Could you check a few things on this model? Use its own coordinates, in mm. Face numbers are marked on the shaded views. A direction names the side the tool comes from. Coordinates: 2 decimals unless noted, no trailing zeros. Loops run counter-clockwise (first coordinate to the right, second up) from the corner with the lowest first, then second, coordinate; pieces in that order, holes last. Notation, with made-up numbers: (49.5, -32) - (101.5, -32) arc R24 cw to (101.5, 4) - close; hole circle Ø9 at (29.25, 66.5). An arc over 180 degrees is marked (long way). Use CSV: the item, a comma, the result in double quotes.
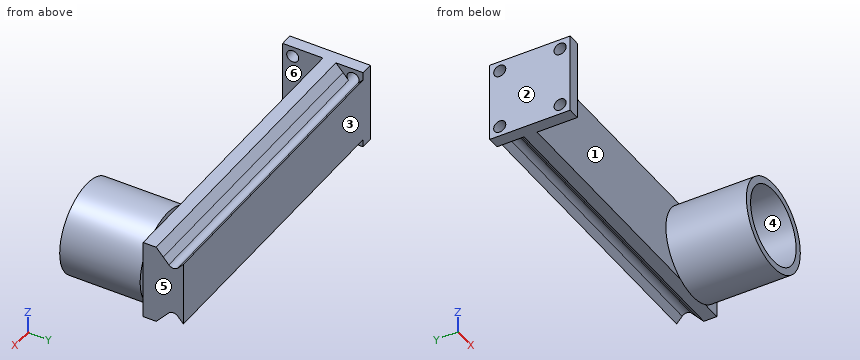
Autodesk Inventor part; units mm, degrees
ref_plane "Work Plane4" through (0, 0, 20) normal (0, 0, -1) x (1, 0, 0)
ref_plane "YZ Plane" through (0, 0, 0) normal (1, 0, 0) x (0, 1, 0)
ref_plane "XZ Plane" through (0, 0, 0) normal (0, 1, 0) x (-1, 0, 0)
sketch "Sketch1" plane through (0, 0, 0) normal (1, 0, 0) x (0, 1, 0)
  line L0 (-20, 20) -> (20, 20)
  line L1 (20, 20) -> (20, -20)
  line L2 (20, -20) -> (-20, -20)
  line L3 (-20, -20) -> (-20, 20)
  line L4 (-20, 20) -> (20, -20) construction
  line L5 (20, 20) -> (-20, -20) construction
  point P0 (0, 0)
  dimension "d0" = 40
  dimension "d1" = 40
extrude "Extrusion1" add sketch "Sketch1" along normal mid plane 6
sketch "Sketch2" plane through (3, 0, 0) normal (1, 0, 0) x (0, 0, -1)
  line L0 (20, 20) -> (-20, 20)
  line L1 (-20, 20) -> (-15, 20)
  line L2 (-15, 20) -> (-15, 15)
  line L3 (-15, 15) -> (-20, 15)
  line L4 (-20, 20) -> (-20, -20)
  circle A0 centre (-15, 15) radius 3
  point P0 (0, 0)
  dimension "d4" = 5
  dimension "d5" = 5
  dimension "d6" = 6
extrude "Extrusion2" cut sketch "Sketch2" against normal blind 6 contours A0 L3 L2 | L2 L3 A0
mirror "Mirror1" about plane through (0, 0, 0) normal (0, 0, 1) of "Extrusion2"
mirror "Mirror2" about plane through (0, 0, 0) normal (0, 1, 0) of "Extrusion2", "Mirror1"
ref_plane "Work Plane4" through (0, 0, 20) normal (0, 0, -1) x (1, 0, 0)
ref_plane "Work Plane3" through (0, 0, 0) normal (0, 0, -1) x (1, 0, 0)
sketch "Sketch3" plane through (0, 0, 20) normal (0, 0, -1) x (1, 0, 0)
  line L0 (3, -20) -> (3, 20)
  line L1 (3, 0) -> (3, -15)
  line L2 (3, -15) -> (153, -15) construction
  line L3 (3, 0) -> (3, -7.5)
  point P0 (0, 0)
  dimension "d10" = 15
  dimension "d11" = 150
  dimension "d12" = 7.5
sketch "Sketch4" plane through (3, 0, 0) normal (1, 0, 0) x (0, 0, -1)
  circle A0 centre (-15, 15) radius 3
  circle A1 centre (15, 15) radius 3
  circle A2 centre (-15, 15) radius 3
  circle A3 centre (-15, 15) radius 3
  circle A4 centre (15, 15) radius 3
  line L0 (-20, 20) -> (20, 20)
  line L1 (-16.0857, 20) -> (-12.9984, 17.2346)
  line L2 (-17.7822, 15) -> (18, 15)
  circle A5 centre (15, 15) radius 3
  line L3 (-16.0857, 10) -> (-12.9984, 12.7654)
  line L4 (0, 20) -> (0, 0)
  line L5 (-16.0857, 10) -> (-20, 6.4938)
  line L6 (-20, -20) -> (-20, 20)
  line L7 (-20, 6.4938) -> (-20, 0)
  circle A6 centre (15, 15) radius 3
  line L8 (16.0857, 20) -> (12.9984, 17.2346)
  line L9 (16.0857, 10) -> (12.9984, 12.7654)
  line L10 (16.0857, 10) -> (20, 6.4938)
  line L11 (20, 6.4938) -> (20, 0)
  line L12 (-16.0857, 20) -> (16.0857, 20)
  line L13 (-20, 0) -> (20, 0)
extrude "Extrusion3" add sketch "Sketch4" along normal blind 150 contours L2 L4 L13 L6 L5 L3 A0 | A0 L1 L0 L4 L2 | L4 L0 L8 A1 L2 | L2 A1 L9 L10 L11 L13 L4
sketch "Sketch5" plane through (3, 0, -20) normal (0, -1, 0) x (1, 0, 0)
  line L0 (150, 0) -> (150, 40)
  line L1 (150, 40) -> (150, 50)
  line L2 (150, 50) -> (150, -10)
  line L3 (150, 3.9143) -> (150, 36.0857)
  line L4 (150, 20) -> (110, 20)
  circle A0 centre (130, 20) radius 22.5
  point P0 (-3, 20)
  dimension "d15" = 10
  dimension "d16" = 60
  dimension "d17" = 40
  dimension "d18" = 45
extrude "Extrusion4" add sketch "Sketch5" along normal blind 40
sketch "Sketch6" plane through (133, -40, 0) normal (0, -1, 0) x (1, 0, 0)
  circle A0 centre (0, 0) radius 19
  point P0 (-133, 0)
  dimension "d21" = 38
extrude "Extrusion5" cut sketch "Sketch6" against normal blind 25
ref_plane "Work Plane1" through (0, 0, 0) normal (0, 0, 1) x (1, 0, 0)
ref_plane "Work Plane2" through (0, 0, 0) normal (0, 0, -1) x (1, 0, 0)
properties part number "TopBracket"
(1) Please list where these lines run through material, in increasing order: line 1 (Y direction, x = 0.85, z = 15); line 2 (X direction, y = -36.5, z = -1).
Computed:
line 1,"y = -20 to -18, -12 to 12, 18 to 20"
line 2,"x = 110.52 to 114.03, 151.97 to 155.48"
(2) Will these pins go through, and if not, where does the flat tip stop? pin 1 (6.5 mm diameter, centred on x = -1, z = -0.5, fed in from -Y); pin 2 (12 mm diameter, centred on x = 44, y = -3.5, fed in from -Z); pin 3 (10 mm diameter, centred on y = 9.5, z = 9, fed in from +X).
Computed:
pin 1,"stops at y = -20"
pin 2,"stops at z = -20"
pin 3,"stops at x = 153"
(3) Thinking about a two-plate mould opening in X: for the marked faces 1, 2 and 3, which applies, +X half, -X half, draft (parallel to the pull), parting line (faces both ways), or undercut?
Computed:
face 1,"undercut"
face 2,"-X half"
face 3,"draft"
(4) Suppose I cut it at B-B (z = 0). Write out the boundary of the cut face in (x, y), plus the area to 3 significant figures.
Computed:
outline,"(-3, -20) - (3, -20) - (3, 0) - (110.5, 0) - (110.5, -40) - (114, -40) - (114, -15) - (152, -15) - (152, -40) - (155.5, -40) - (155.5, 0) - (153, 0) - (153, 20) - (-3, 20) - close"
area,"4,090 mm²"
(5) Suppose I cut it at C-C (x = 137.5). Write out the boundary of the cut face in (y, z).
Computed:
outline,"(-40, -22.05) - (0, -22.05) - (0, -20) - (6.49, -20) - (10, -16.09) - (12.77, -13) arc R3 cw to (17.23, -13) - (20, -16.09) - (20, 16.09) - (17.23, 13) arc R3 cw to (12.77, 13) - (10, 16.09) - (6.49, 20) - (0, 20) - (0, 22.05) - (-40, 22.05) - (-40, 18.46) - (-15, 18.46) - (-15, -18.46) - (-40, -18.46) - close"
(6) Suppose I cut it at D-D (x = 44.5). Write out the boundary of the cut face in (y, z).
Computed:
outline,"(0, -20) - (6.49, -20) - (10, -16.09) - (12.77, -13) arc R3 cw to (17.23, -13) - (20, -16.09) - (20, 16.09) - (17.23, 13) arc R3 cw to (12.77, 13) - (10, 16.09) - (6.49, 20) - (0, 20) - close"
(7) Which directions (+Z, -Z, +X, -X, +Y, -Y) give clear straight access to the entire face, cutting with the end or side of a thin tool? Please do the marked faces 4, 5 and 6.
Computed:
face 4,"-Y"
face 5,"+Z, -Z, +X, +Y"
face 6,"+Z, -Z, -Y"
(8) Suppose I cut it at A-A (y = -24). Write out the boundary of the cut face in (x, z).
Computed:
outline,"circle Ø45 at (133, 0); hole circle Ø38 at (133, 0)"
